Design review of the part built by this model. Coordinates are the model's own, in mm. Coordinates: 2 decimals unless noted, no trailing zeros. Write each loop counter-clockwise with the first axis right and the second up, starting at its lowest first coordinate (ties: lowest second). Pieces come first, ordered by that corner, then holes.
Q1. For L1, parallel to Y at x = 35, z = 2.15; L2, parallel to X at y = 5.25, z = 1.05; L3, parallel to X at y = 6, z = 0.45 (3 decimals), list the stretches that pass through material, from the lowest coordinate up.
Q2. Take a section at B-B, the plane z = 1.55. Write out the cut boundary in (x, y), plus the area to 3 significant figures.
Q3. Take a section at C-C, the plane y = 5. Write out the cut boundary in (x, z), plus the area to 3 significant figures.
Q4. Take a section at A-A, the plane x = 35. Write out the cut boundary in (y, z).
from build123d import *

# Parameters (mm, degrees)
SKETCH1_W             = 80
SKETCH1_H             = 10
SKETCH1_R             = 1.300963213
BOSS_EXTRUDE1_DEPTH   = 3
M3_TAPPED_HOLE1_D     = 2.5
M3_TAPPED_HOLE1_DEPTH = 7.5
M3_TAPPED_HOLE1_TIP   = 0.751075774


with BuildPart() as part:
    # Sketch1 → Boss-Extrude1 (new body)
    with BuildSketch(Plane.XY):
        with Locations((71.266417393, 5)):
            Rectangle(SKETCH1_W, SKETCH1_H)
        with Locations((35, 5)):
            Circle(SKETCH1_R, mode=Mode.SUBTRACT)
        with Locations(Location((107.532834786, 5, 0), (0, 0, 180))):
            Circle(SKETCH1_R, mode=Mode.SUBTRACT)
    extrude(amount=BOSS_EXTRUDE1_DEPTH)

    # M3 Tapped Hole1
    with Locations(Plane.XY.offset(3)):
        with Locations((99.532834786, 5)):
            Hole(M3_TAPPED_HOLE1_D / 2, depth=M3_TAPPED_HOLE1_DEPTH)
            with Locations((0, 0, -(M3_TAPPED_HOLE1_DEPTH + M3_TAPPED_HOLE1_TIP / 2))):  # 118° drill point
                Cone(0, M3_TAPPED_HOLE1_D / 2, M3_TAPPED_HOLE1_TIP, mode=Mode.SUBTRACT)


solid = part.part
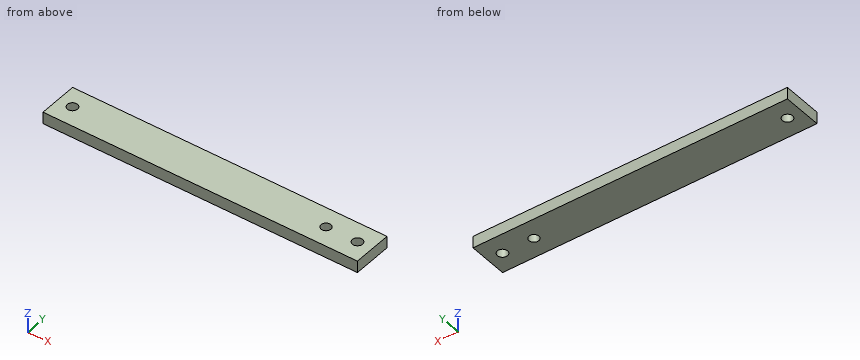
Responses:
1. L1: y = 0 to 3.7, 6.3 to 10
1. L2: x = 31.27 to 33.72, 36.28 to 98.31, 100.76 to 106.26, 108.81 to 111.27
1. L3: x = 31.266 to 34.168, 35.832 to 98.783, 100.283 to 106.701, 108.365 to 111.266
2. outline: (31.27, 0) - (111.27, 0) - (111.27, 10) - (31.27, 10) - close; hole circle Ø2.6 at (35, 5); hole circle Ø2.5 at (99.53, 5); hole circle Ø2.6 at (107.53, 5)
2. area: 784 mm2
3. outline: (31.27, 0) - (33.7, 0) - (33.7, 3) - (31.27, 3) - close; (36.3, 0) - (98.28, 0) - (98.28, 3) - (36.3, 3) - close; (100.78, 0) - (106.23, 0) - (106.23, 3) - (100.78, 3) - close; (108.83, 0) - (111.27, 0) - (111.27, 3) - (108.83, 3) - close
3. area: 217 mm2
4. outline: (0, 0) - (3.7, 0) - (3.7, 3) - (0, 3) - close; (6.3, 0) - (10, 0) - (10, 3) - (6.3, 3) - close
